from build123d import *

# Parameters (mm, degrees)
BEARING_START             = 1
SKETCH1_R                 = 25
SKETCH1_R_2               = 22
BEARING_RING_INSERT_DEPTH = 7
SKETCH2_R                 = 22
BULK_EXTRUDE_DEPTH        = 3


with BuildPart() as part:
    # Sketch1 → BEARING RING INSERT (new body)
    with BuildSketch(Plane(origin=(74, 0, 0), x_dir=(0, 0, -1), z_dir=(1, 0, 0)).offset(BEARING_START)):
        with Locations((50, -18.372727273)):
            Circle(SKETCH1_R)
        with Locations((50, -18.372727273)):
            Circle(SKETCH1_R_2, mode=Mode.SUBTRACT)
    extrude(amount=BEARING_RING_INSERT_DEPTH)

    # Sketch2 → BULK EXTRUDE (add)
    with BuildSketch(Plane(origin=(82, 0, 0), x_dir=(0, 0, -1), z_dir=(1, 0, 0))):
        with BuildLine():
            Line((105, -18.372727273), (105, 69.627272727))
            Line((105, 69.627272727), (-5, 69.627272727))
            Line((-5, 69.627272727), (-5, -18.372727273))
            ThreePointArc((-5, -18.372727273), (50, -73.372727273), (105, -18.372727273))
        make_face()
        with Locations((50, -18.372727273)):
            Circle(SKETCH2_R, mode=Mode.SUBTRACT)
    extrude(amount=BULK_EXTRUDE_DEPTH)


solid = part.part
Model file for the job. Use its own axes, mm. A direction names the side the tool comes from. Coordinates: 2 decimals unless noted, no trailing zeros. Order: outer loops, then holes, each group sorted by start corner. A loop starts at its lowest first (then second) coordinate and runs counter-clockwise, first axis right, second up. Notation, with made-up numbers: (-4.75, 71.25) -> (22.25, 71.25) arc R21 ccw to (22.25, 103.25) -> close; hole circle Ø2 at (53, -6). An arc over 180 degrees is marked (long way). Return JSON: item names as keys, results as strings. Group by question number.
Item 1: Saw through at B-B on x = 83.5. Write the cut outline in (y, z).
Item 2: Saw through at D-D on z = -32.5. Write the cut outline in (x, y), then the cut area to 3 significant figures.
Item 3: Pull direction Z, two halves, no side cores. Call faces 3 (the flat face through (85, 15, -49)), 4 (the flat face through (83, 26, 5)), 5 (the cylindrical face through (79.93, -26.8, -70.32)): pulls with the +Z half, pulls with the -Z half, needs draft (parallel to the pull), parting line crosses it, or undercut.
Item 4: Tool access for faces 1 (the flat face through (82, 15, -49)), 2 (the flat face through (75, -40.5, -51.7)): list every direction of +Z, -Z, +X, -X, +Y, -Y with a clear straight run to the whole face (end or side of a thin tool).
Item 5: Saw through at C-C on y = 54.5. Write the cut outline in (x, z), then the cut area to 3 significant figures.
Item 6: Wall check: line 1 along Y through (x, z) = (80, -50); line 2 along X through (y, z) = (49, -8); line 3 along Z through (x, y) = (78, 1.5). Give the ranges that are in metal, low to high. Write a range as [from, to].
Item 7: Flat gauge pins, fed straight in: P1, Ø5, axis at x = 80.5, y = 49.5, coming from the +Z side; P2, Ø1.5, axis at x = 83, y = -57, coming from the -Z side; P3, Ø2, axis at x = 76, z = -67, coming from the +Y side. Where does each tip first touch, or does it go through?
Item 8: Saw through at A-A on z = -50. Write the cut outline in (x, y), then the cut area to 3 significant figures.
Values found:
{
 "1": {"outline": "(-18.37, -105) -> (69.63, -105) -> (69.63, 5) -> (-18.37, 5) arc R55 ccw to start; hole circle Ø44 at (-18.37, -50)"},
 "2": {"outline": "(75, -36.23) -> (82, -36.23) -> (82, -70.51) -> (85, -70.51) -> (85, -31.71) -> (75, -31.71) -> close; (75, -5.04) -> (85, -5.04) -> (85, 69.63) -> (82, 69.63) -> (82, -0.52) -> (75, -0.52) -> close", "area": "404 mm2"},
 "3": {"face 3": "needs draft", "face 4": "pulls with the +Z half", "face 5": "undercut"},
 "4": {"face 1": "-X", "face 2": "+Z, -Z, -X, +Y, -Y"},
 "5": {"outline": "(82, -105) -> (85, -105) -> (85, 5) -> (82, 5) -> close", "area": "330 mm2"},
 "6": {"line 1": "y = [-43.37, -40.37], [3.63, 6.63]", "line 2": "x = [82, 85]", "line 3": "z = [-65.17, -59.44], [-40.56, -34.83]"},
 "7": {"P1": "stops at z = 5", "P2": "stops at z = -89.88", "P3": "stops at y = 0.84"},
 "8": {"outline": "(75, -43.37) -> (82, -43.37) -> (82, -73.37) -> (85, -73.37) -> (85, -40.37) -> (75, -40.37) -> close; (75, 3.63) -> (85, 3.63) -> (85, 69.63) -> (82, 69.63) -> (82, 6.63) -> (75, 6.63) -> close", "area": "339 mm2"}
}
